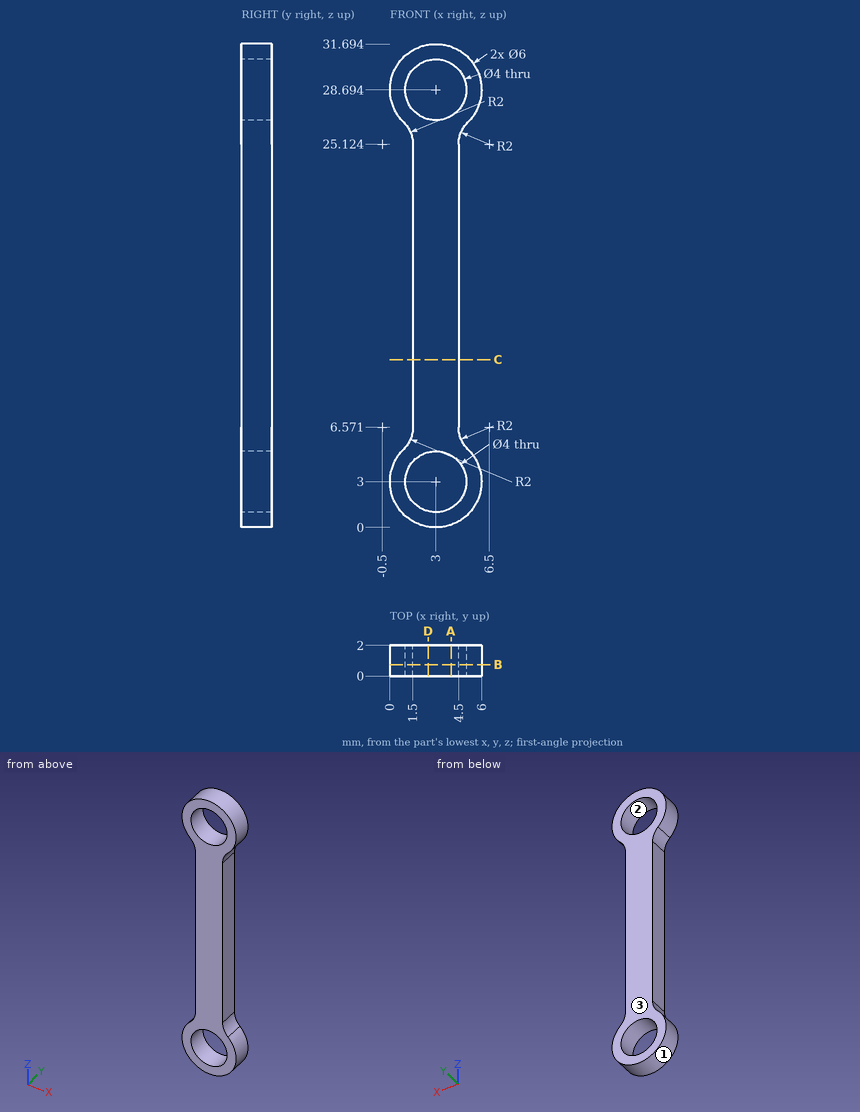
Job drawing, mm, ordinate dimensions from the low corner. One solid piece. Coordinates: 2 decimals unless noted, no trailing zeros. Loops run counter-clockwise (first coordinate to the right, second up) from the corner with the lowest first, then second, coordinate; pieces in that order, holes last. Notation, with made-up numbers: (55.5, 38) - (88.5, 38) arc R16 ccw to (88.5, 44) - close; hole circle Ø6 at (6.25, 82.5). An arc over 180 degrees is marked (long way). Write item = value, one per line. Start each with the question number.
Q1. Flat gauge pins, fed straight in: pin 1 Ø1.5 at (x, z) = (5, 16.5) entering from -Y; pin 2 Ø0.6 at (y, z) = (1.5, 12.5) entering from +X; pin 3 Ø3 at (x, z) = (3, 3) entering from -Y; pin 4 Ø1 at (y, z) = (1, 17.5) entering from -X. Where does each tip first touch, or does it go through?
Q2. Cut at A-A, the plane x = 4. List the corners of the cut face in (y, z).
Q3. Cut at D-D, the plane x = 2.5. List the corners of the cut face in (y, z).
Q4. Pull direction X, two halves, no side cores. Call the marked faces 1, 2 and 3: pulls with the +X half, pulls with the -X half, needs draft (parallel to the pull), parting line crosses it, or undercut.
Q5. Drill centre lines: L1, parallel to Z at x = 3.25, y = 0.15 (1 decimal); L2, parallel to Z at x = 4, y = 1.4 (1 decimal); L3, parallel to X at y = 1, z = 21. Where is each one in solid material? Low to high.
Q6. Cut at C-C, the plane z = 11. List the corners of the cut face in (x, y).
Q7. Cut at B-B, the plane y = 0.75. List the corners of the cut face in (x, z) (1 decimal).
Computed:
q1.pin_1 = 0
q1.pin_2 = 4.5
q1.pin_3 = through
q1.pin_4 = 1.5
q2.outline = (0, 0.17) - (2, 0.17) - (2, 1.27) - (0, 1.27) - close; (0, 4.73) - (2, 4.73) - (2, 26.96) - (0, 26.96) - close; (0, 30.43) - (2, 30.43) - (2, 31.52) - (0, 31.52) - close
q3.outline = (0, 0.04) - (2, 0.04) - (2, 1.06) - (0, 1.06) - close; (0, 4.94) - (2, 4.94) - (2, 26.76) - (0, 26.76) - close; (0, 30.63) - (2, 30.63) - (2, 31.65) - (0, 31.65) - close
q4.face_1 = parting line crosses it
q4.face_2 = undercut
q4.face_3 = needs draft
q5.L1 = 0 to 1, 5 to 26.7, 30.7 to 31.7
q5.L2 = 0.2 to 1.3, 4.7 to 27, 30.4 to 31.5
q5.L3 = 1.5 to 4.5
q6.outline = (1.5, 0) - (4.5, 0) - (4.5, 2) - (1.5, 2) - close
q7.outline = (0.9, 5.1) arc R3 ccw (long way) to (5.1, 5.1) arc R2 cw to (4.5, 6.6) - (4.5, 25.1) arc R2 cw to (5.1, 26.6) arc R3 ccw (long way) to (0.9, 26.6) arc R2 cw to (1.5, 25.1) - (1.5, 6.6) arc R2 cw to start; hole circle Ø4 at (3, 3); hole circle Ø4 at (3, 28.7)
